```python
from build123d import *

# Parameters (mm, degrees)
SKETCH1_R           = 17.5
BOSS_EXTRUDE1_DEPTH = 8
CUT_EXTRUDE1_DEPTH  = 9
CUT_EXTRUDE2_DEPTH  = 10
CIRPATTERN1_COUNT   = 24


with BuildPart() as part:
    # Sketch1 → Boss-Extrude1 (new body)
    with BuildSketch(Plane(origin=(0, 0, 0), x_dir=(1, 0, 0), z_dir=(0, 1, 0))):
        Circle(SKETCH1_R)
    extrude(amount=BOSS_EXTRUDE1_DEPTH)

    # Sketch2 → Cut-Extrude1 (cut, through all)
    with BuildSketch(Plane(origin=(0, 8, 0), x_dir=(1, 0, 0), z_dir=(0, 1, 0))):
        with BuildLine():
            Line((-1.88867937, 0.797113692), (1.88867937, 0.797113692))
            ThreePointArc((1.88867937, 0.797113692), (0, -2.05), (-1.88867937, 0.797113692))
        make_face()
    extrude(amount=-CUT_EXTRUDE1_DEPTH, mode=Mode.SUBTRACT)

    # Sketch3 → Cut-Extrude2 (cut)
    with BuildSketch(Plane(origin=(0, 8, 0), x_dir=(1, 0, 0), z_dir=(0, 1, 0))):
        Polygon((0, 14), (0.6, 14), (1.8, 17.407182426), (1.8, 19.314701451), (-1.8, 19.314701451), (-1.8, 17.407182426), (-0.6, 14), align=None)
    cut_extrude2 = extrude(amount=-CUT_EXTRUDE2_DEPTH, mode=Mode.SUBTRACT)

    # CirPattern1: Cut-Extrude2 ×24 about axis
    cirpattern1_axis = Axis((0, 0, 0), (0, 1, 0))
    for i in range(1, CIRPATTERN1_COUNT):
        add(cut_extrude2.rotate(cirpattern1_axis, i * 360 / CIRPATTERN1_COUNT), mode=Mode.SUBTRACT)


solid = part.part
```
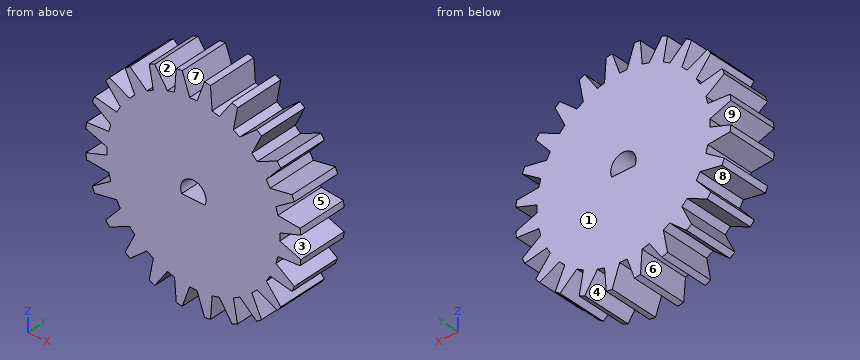
For this review, take the finished solid that the model builds, in its own axes (mm). Face numbers are marked on the shaded views. A direction names the side the tool comes from. Give positions to 0.01 mm unless a question says otherwise; leave off trailing zeros. Loops run counter-clockwise (first coordinate to the right, second up) from the corner with the lowest first, then second, coordinate; pieces in that order, holes last. Notation, with made-up numbers: M 43,78.5 L 67,78.5 A19 ccw 67,109.5 Z; hole C 57.25,58.5 d7. An arc over 180 degrees is marked long. One line per item, written item: value. Start each with the question number.
Q1. Add section D-D (z = -5.5). Give the boundary of the cut face in (x, y), and give its area (3 significant figures).
Q2. Add section A-A (z = 0). Give the boundary of the cut face in (x, y), and give its area (3 significant figures).
Q3. Add section C-C (z = 8.5). Give the boundary of the cut face in (x, y).
Q4. Machinability: for the marked faces 5, 6, 7, 8 and 9, which of the approach directions +Z, -Z, +X, -X, +Y, -Y give a long, thin tool a straight path to every point of the face, cutting with its end or side? Answer none if there is none.
Q5. Add section B-B (x = 0). Give the boundary of the cut face in (y, z), and give its area (3 significant figures).
Q6. Clearance check with flat-ended pins moving along their axes: pin 1 Ø1 at (y, z) = (5.5, 0) entering from +X; pin 2 Ø4 at (y, z) = (2, 5) entering from -X. State where each tip first meets the part, or that it passes through.
Q7. Draft analysis for pull direction Z (two halves, no side actions). For the marked faces 1, 2, 3 and 4, state which applies: released by +Z, released by -Z, zero draft, split by the parting line, or undercut.
Q8. For L1, parallel to X at y = 2, z = 0; L2, parallel to X at y = 3.5, z = -15; L3, parallel to X at y = 6.75, z = 12.5, list the stretches that pass through material, from the lowest coordinate up.
Reply:
1. outline: M -15.26,0 L 15.26,0 L 15.26,8 L -15.26,8 Z
1. area: 244 mm²
2. outline: M -14,0 L -2.05,0 L -2.05,8 L -14,8 Z; M 2.05,0 L 14,0 L 14,8 L 2.05,8 Z
2. area: 191 mm²
3. outline: M -12.66,0 L 12.66,0 L 12.66,8 L -12.66,8 Z
4. face 5: +X, +Y, -Y
4. face 6: -Z, +Y, -Y
4. face 7: +Z, +Y, -Y
4. face 8: +Y, -Y
4. face 9: -X, +Y, -Y
5. outline: M 0,-14 L 8,-14 L 8,-0.8 L 0,-0.8 Z; M 0,2.05 L 8,2.05 L 8,14 L 0,14 Z
5. area: 201 mm²
6. pin 1: x = 14
6. pin 2: x = -16.35
7. face 1: zero draft
7. face 2: released by +Z
7. face 3: undercut
7. face 4: released by -Z
8. L1: -14 to -2.05, 2.05 to 14
8. L2: -6.96 to -5.32, -2.94 to -0.95, 0.95 to 2.94, 5.32 to 6.96
8. L3: -10.52 to -8.31, -6.49 to 6.49, 8.31 to 10.52
